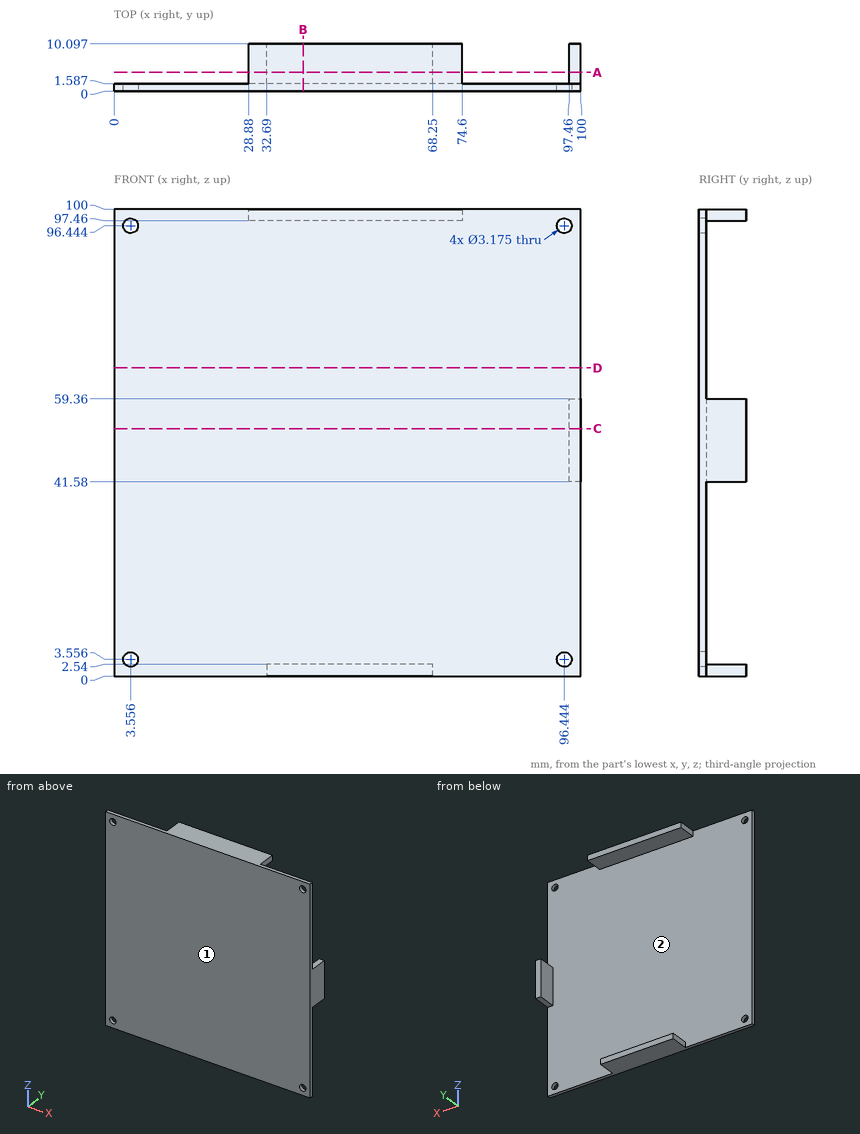
The figure shows three views and two pictorial views of one solid part (mm, origin at its lowest corner). Answer the questions. Give positions to 0.01 mm unless a question says otherwise; leave off trailing zeros. Write each loop counter-clockwise with the first axis right and the second up, starting at its lowest first coordinate (ties: lowest second). Pieces come first, ordered by that corner, then holes. Notation, with made-up numbers: M -37,3.5 L -15,3.5 A31 cw -15,35.5 Z; hole C 59,32 d4. An arc over 180 degrees is marked long. One line per item, written item: value. Start each with the question number.
(1) Find section D-D (z = 66). Determine the outline of the cut face in (x, y), plus the area to 3 significant figures.
(2) Determine the mould class of the marked faces 1 and 2 for opening direction Z: pulls with the +Z half, pulls with the -Z half, needs draft (parallel to the pull), parting line crosses it, or undercut.
(3) Find the intervals of material crossed by line 1 (Z direction, x = 34.5, y = 8.5); line 2 (Y direction, x = 55.5, z = 27); line 3 (X direction, y = 3.5, z = 53.5), in increasing order.
(4) Flat-ended cylindrical pins translate along their axes: pin 1 Ø2 at (x, z) = (36.5, 78) entering from -Y; pin 2 Ø3 at (x, y) = (99, 5) entering from +Z; pin 3 Ø2 at (y, z) = (5.5, 0.5) entering from -X; pin 4 Ø0.8 at (y, z) = (7.5, 1) entering from +X. Find the tip coordinate at first contact, or state that the pin passes through.
(5) Find section A-A (y = 4). Determine the outline of the cut face in (x, z).
(6) Find section B-B (x = 40.5). Determine the outline of the cut face in (y, z).
(7) Find section C-C (z = 53). Determine the outline of the cut face in (x, y).
Results below:
1. outline: M 0,0 L 100,0 L 100,1.59 L 0,1.59 Z
1. area: 159 mm^2
2. face 1: needs draft
2. face 2: undercut
3. line 1: z = 0 to 2.54, 97.46 to 100
3. line 2: y = 0 to 1.59
3. line 3: x = 97.46 to 100
4. pin 1: stops at y = 0
4. pin 2: stops at z = 59.36
4. pin 3: stops at x = 32.69
4. pin 4: stops at x = 68.25
5. outline: M 28.88,97.46 L 74.6,97.46 L 74.6,100 L 28.88,100 Z; M 32.69,0 L 68.25,0 L 68.25,2.54 L 32.69,2.54 Z; M 97.46,41.58 L 100,41.58 L 100,59.36 L 97.46,59.36 Z
6. outline: M 0,0 L 10.1,0 L 10.1,2.54 L 1.59,2.54 L 1.59,97.46 L 10.1,97.46 L 10.1,100 L 0,100 Z
7. outline: M 0,0 L 100,0 L 100,10.1 L 97.46,10.1 L 97.46,1.59 L 0,1.59 Z
